Part model, mm, in its own coordinate system. A direction names the side the tool comes from. Give positions to 0.01 mm unless a question says otherwise; leave off trailing zeros. Write each loop counter-clockwise with the first axis right and the second up, starting at its lowest first coordinate (ties: lowest second). Pieces come first, ordered by that corner, then holes.
```python
from build123d import *

# Parameters (mm, degrees)
F0_W     = 8.368255198
F0_H     = 8.1290510939
F1_DEPTH = 5
F2_DEPTH = 25


with BuildPart() as f1:
    # F0 (on Top) → F1 (new body)
    with BuildSketch(Plane.XY):
        with Locations((-20.815872401, 12.7671566554)):
            Rectangle(F0_W, F0_H)
        Polygon((16.631744802, 16.8316822024), (-16.631744802, 16.8316822024), (-16.631744802, 8.7026311085), (-25, 8.7026311085), (-25, -8.7026311085), (-16.631744802, -8.7026311085), (-16.631744802, -16.8316822024), (16.631744802, -16.8316822024), (16.631744802, -8.7026311085), (25, -8.7026311085), (25, 8.7026311085), (16.631744802, 8.7026311085), align=None)
        with Locations((20.815872401, 12.7671566554)):
            Rectangle(F0_W, F0_H)
        with Locations((-20.815872401, -12.7671566554)):
            Rectangle(F0_W, F0_H)
        with Locations((20.815872401, -12.7671566554)):
            Rectangle(F0_W, F0_H)
    extrude(amount=F1_DEPTH)

    # F0 (on Top) → F2 (join)
    with BuildSketch(Plane.XY):
        with Locations((20.815872401, 12.7671566554)):
            Rectangle(F0_W, F0_H)
        with Locations((20.815872401, -12.7671566554)):
            Rectangle(F0_W, F0_H)
        with Locations((-20.815872401, -12.7671566554)):
            Rectangle(F0_W, F0_H)
        with Locations((-20.815872401, 12.7671566554)):
            Rectangle(F0_W, F0_H)
    extrude(amount=F2_DEPTH)


solid = f1.part
```
1) Two-plate mould, pull along Y, no slides. Class faces 1 (the face through (21, -8.703, 15)), 2 (the face through (-6, -16.832, 4)), 3 (the face through (-16.632, -13, 15)): +Y half, -Y half, draft (parallel to the pull), parting line (faces both ways), or undercut.
Answers follow:
face 1: undercut
face 2: -Y half
face 3: draft
2) Pin check, flat tip, straight feed: pin 1 Ø10 at (x, y) = (4, 7) entering from +Z. Stop position of the tip, or through.
Answers follow:
pin 1: stops at z = 5
3) Saw through at C-C, the plane x = -21.5. Write the cut outline in (y, z).
Answers follow:
outline: (-16.83, 0) - (16.83, 0) - (16.83, 25) - (8.7, 25) - (8.7, 5) - (-8.7, 5) - (-8.7, 25) - (-16.83, 25) - close
4) Saw through at D-D, the plane x = -14.5. Write the cut outline in (y, z), then the cut area to 3 significant figures.
Answers follow:
outline: (-16.83, 0) - (16.83, 0) - (16.83, 5) - (-16.83, 5) - close
area: 168 mm2
5) Saw through at A-A, the plane z = 15.25. Write the cut outline in (x, y).
Answers follow:
outline: (-25, -16.83) - (-16.63, -16.83) - (-16.63, -8.7) - (-25, -8.7) - close; (-25, 8.7) - (-16.63, 8.7) - (-16.63, 16.83) - (-25, 16.83) - close; (16.63, -16.83) - (25, -16.83) - (25, -8.7) - (16.63, -8.7) - close; (16.63, 8.7) - (25, 8.7) - (25, 16.83) - (16.63, 16.83) - close
6) 3-axis set-ups, long thin cutter, end or side, ignore diameter. For faces 4 (the face through (-21, -13, 25)), 5 (the face through (16.632, -13, 15)), 6 (the face through (-21, 8.703, 15)): which of +Z, -Z, +X, -X, +Y, -Y reach the whole face in a straight line?
Answers follow:
face 4: +Z, +X, -X, +Y, -Y
face 5: +Z, +Y, -Y
face 6: +Z, +X, -X
7) Wall check: L1, parallel to X at y = 15.5, z = 21.5; L2, parallel to Y at x = 21.5, z = 17.5; L3, parallel to Z at x = 9, y = -3.5. Give the ranges that are in metal, low to high.
Answers follow:
L1: x = -25 to -16.63, 16.63 to 25
L2: y = -16.83 to -8.7, 8.7 to 16.83
L3: z = 0 to 5
8) Saw through at B-B, the plane y = 12. Write the cut outline in (x, z), then the cut area to 3 significant figures.
Answers follow:
outline: (-25, 0) - (25, 0) - (25, 25) - (16.63, 25) - (16.63, 5) - (-16.63, 5) - (-16.63, 25) - (-25, 25) - close
area: 585 mm2
